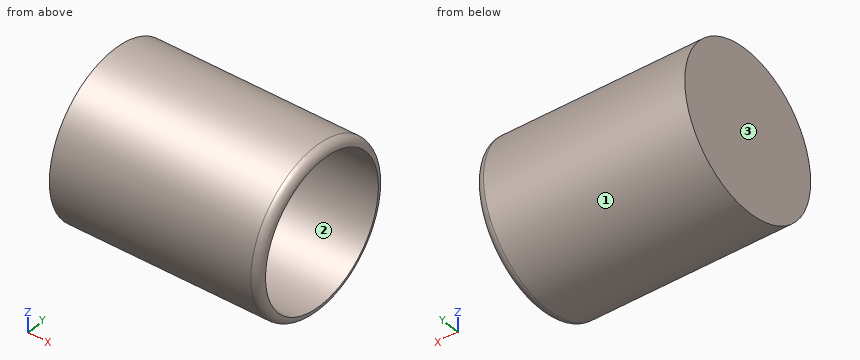
```python
from build123d import *

# Parameters (mm, degrees)
F0_R     = 49.3246068697
F1_DEPTH = 127
F2_R     = 5.08
F3_DEPTH = 25.4
F4_DEPTH = 25.4
F5_DEPTH = 25.4
F6_DEPTH = 25.4


with BuildPart() as f1:
    # F0 (on Right) → F1 (new body)
    with BuildSketch(Plane.YZ):
        Circle(F0_R)
    extrude(amount=F1_DEPTH)

    # F2
    f2_edges = [f1.edges().sort_by_distance(p)[0] for p in [
        (127, -49.324607, 0),
    ]]
    fillet(f2_edges, radius=F2_R)

    # F3 (cut): a face of the model
    f3_faces = [f1.faces().sort_by_distance(p)[0] for p in [
        (127, 0, 0),
    ]]
    extrude(f3_faces, amount=-F3_DEPTH, mode=Mode.SUBTRACT)

    # F4 (cut): a face of the model
    f4_faces = [f1.faces().sort_by_distance(p)[0] for p in [
        (101.6, 0, 0),
    ]]
    extrude(f4_faces, amount=-F4_DEPTH, mode=Mode.SUBTRACT)

    # F5 (cut): a face of the model
    f5_faces = [f1.faces().sort_by_distance(p)[0] for p in [
        (76.2, 0, 0),
    ]]
    extrude(f5_faces, amount=-F5_DEPTH, mode=Mode.SUBTRACT)

    # F6 (cut): a face of the model
    f6_faces = [f1.faces().sort_by_distance(p)[0] for p in [
        (50.8, 0, 0),
    ]]
    extrude(f6_faces, amount=-F6_DEPTH, mode=Mode.SUBTRACT)


solid = f1.part
```
Can you work these out from the model? Positions are in its coordinate system, mm. Face numbers are marked on the shaded views. Coordinates: 2 decimals unless noted, no trailing zeros. Order: outer loops, then holes, each group sorted by start corner. A loop starts at its lowest first (then second) coordinate and runs counter-clockwise, first axis right, second up. Notation, with made-up numbers: (55, -1) -> (65, -1) arc R5 ccw to (65, 8) -> close; hole circle Ø7 at (-19, -3.5). An arc over 180 degrees is marked (long way). Write each question's results on one line, items separated by ' | '.
Item 1: If we mould it in two halves opening along Y, with no side actions, what happens to the marked faces 1, 2 and 3? For each: +Y half, -Y half, draft (parallel to the pull), parting line (faces both ways), or undercut.
Results are:
face 1: parting line | face 2: undercut | face 3: draft
Item 2: I want a section at A-A, the plane z = 0. Write out the boundary of the cut face in (x, y).
Results are:
outline: (0, -49.32) -> (121.92, -49.32) arc R5.08 ccw to (127, -44.24) -> (25.4, -44.24) -> (25.4, 44.24) -> (127, 44.24) arc R5.08 ccw to (121.92, 49.32) -> (0, 49.32) -> close
Item 3: If I drill on line 1 along Z through (x, y) = (46, 0); line 2 along X through (y, z) = (35, 2.5); line 3 along Z through (x, y) = (110, -24), over which ranges is the centre line in solid material (lowest first)?
Results are:
line 1: -49.32 to -44.24, 44.24 to 49.32 | line 2: 0 to 25.4 | line 3: -43.09 to -37.17, 37.17 to 43.09
Item 4: I'm going to push flat-ended pins straight in: pin 1 Ø10 at (x, z) = (49.5, 5.5) entering from -Y; pin 2 Ø4 at (x, y) = (56, 27) entering from -Z; pin 3 Ø6 at (x, z) = (61, 15.5) entering from +Y. Where does each tip first touch, or does it pass through?
Results are:
pin 1: y = -49.32 | pin 2: z = -42.52 | pin 3: y = 47.71
Item 5: I want a section at C-C, the plane x = 105.5. Write out the boundary of the cut face in (y, z).
Results are:
outline: circle Ø98.65 at (0, 0); hole circle Ø88.49 at (0, 0)
Item 6: I want a section at D-D, the plane x = 18. Write out the boundary of the cut face in (y, z), then the cut area to 3 significant figures.
Results are:
outline: circle Ø98.65 at (0, 0) | area: 7,640 mm²
